Design review of the part built by this model. Coordinates are the model's own, in mm. Face numbers are marked on the shaded views. Coordinates: 2 decimals unless noted, no trailing zeros. Write each loop counter-clockwise with the first axis right and the second up, starting at its lowest first coordinate (ties: lowest second). Pieces come first, ordered by that corner, then holes. Notation, with made-up numbers: (-20.75, 82) - (10.25, 82) arc R14 ccw to (10.25, 102) - close; hole circle Ø5 at (87, 78). An arc over 180 degrees is marked (long way). Answer as CSV lines item,"result". Start each with the question number.
Q1. We need section C-C (y = 13). Write out the cut boundary in (x, z).
Q2. We need section A-A (x = -4). Write out the cut boundary in (y, z), plus the area to 3 significant figures.
Q3. We need section B-B (z = 45). Write out the cut boundary in (x, y), plus the area to 3 significant figures.
Q4. Clearance check with flat-ended pins moving along their axes: pin 1 (3.5 mm diameter, centred on y = 5, z = 31, fed in from -X); pin 2 (6.5 mm diameter, centred on x = -2, y = 14, fed in from +Z); pin 3 (0.9 mm diameter, centred on x = -11.5, y = 35.5, fed in from -Z). State where each tip first meets the part, or that it passes through.
Q5. We need section D-D (z = 13). Write out the cut boundary in (x, y).
Q6. Mouldability with a two-part tool opening along Z and no side actions: class the marked faces 1 and 2 as pulls with the +Z half, pulls with the -Z half, needs draft (parallel to the pull), parting line crosses it, or undercut.
Q7. For line 1 along Y through (x, z) = (-8.8, -31); line 2 along Z through (x, y) = (0, 38.1); line 3 along Z through (x, y) = (-2.75, 27), list the stretches that pass through material, from the lowest coordinate up. Write a range as [from, to].
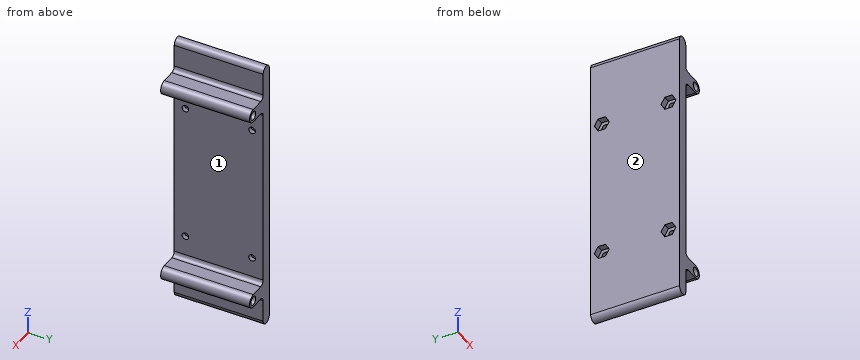
Autodesk Inventor part; units mm, degrees
ref_plane "РабПлоскость1" through (0, 20, 0) normal (0, 1, 0) x (1, 0, 0)
ref_plane "YZ Plane" through (0, 0, 0) normal (1, 0, 0) x (0, 1, 0)
ref_plane "XZ Plane" through (0, 0, 0) normal (0, 1, 0) x (-1, 0, 0)
sketch "Эскиз1" plane through (0, 0, 0) normal (0, 1, 0) x (-1, 0, 0)
  line L0 (0, 45) -> (0, -45) construction
  circle A0 centre (0, 45) radius 1.5
  circle A1 centre (0, -45) radius 1.5
  line L1 (10.5, 60) -> (10.5, -60) construction
  line L2 (10.5, -60) -> (10.5, 60) construction
  line L3 (13, -60) -> (13, 60)
  line L4 (8, 60) -> (8, 48)
  arc A2 (8, -60) -> (13, -60) centre (10.5, -60) ccw
  arc A3 (13, 60) -> (8, 60) centre (10.5, 60) ccw
  arc A4 (0, 42) -> (0, 48) centre (0, 45) ccw construction
  arc A5 (0, -48) -> (0, -42) centre (0, -45) ccw construction
  line L5 (0, 48) -> (8, 48)
  line L6 (0, 42) -> (8, 42)
  line L7 (0, -42) -> (8, -42)
  line L8 (0, -48) -> (8, -48)
  arc A6 (0, -42) -> (0, -48) centre (0, -45) ccw
  arc A7 (0, 48) -> (0, 42) centre (0, 45) ccw
  line L9 (8, -42) -> (8, -48) construction
  line L10 (8, 42) -> (8, -42)
  line L11 (8, -48) -> (8, -60)
  line L12 (8, 48) -> (8, 42) construction
  point P0 (0, 0)
  point P1 (0, 0)
  point P2 (10.5, 0)
  dimension "d0" = 90
  dimension "d1" = 3
  dimension "d2" = 3
  dimension "d3" = 120
  dimension "d4" = 10.5
  dimension "d5" = 0
  dimension "d6" = 5
  dimension "d7" = 6
  dimension "d8" = 6
extrude "Выдавливание1" add sketch "Эскиз1" along normal blind 40
fillet "Сопряжение1" radius 2 4 edges at (-8, 20, 42) (-8, 20, 48) (-8, 20, -42) (-8, 20, -48)
sketch "Эскиз2" plane through (0, 40, 0) normal (0, 1, 0) x (1, 0, 0)
  line L0 (0, 48) -> (-6, 48)
  arc A0 (-8, 50) -> (-6, 48) centre (-6, 50) ccw
  line L1 (-8, 50) -> (-8, 60)
  arc A1 (-8, 60) -> (-13, 60) centre (-10.5, 60) ccw
  line L2 (-13, 60) -> (-13, -60)
  arc A2 (-13, -60) -> (-8, -60) centre (-10.5, -60) ccw
  line L3 (-8, -60) -> (-8, -50)
  arc A3 (-6, -48) -> (-8, -50) centre (-6, -50) ccw
  line L4 (-6, -48) -> (0, -48)
  arc A4 (0, -48) -> (0, -42) centre (0, -45) ccw
  line L5 (0, -42) -> (-6, -42)
  arc A5 (-8, -40) -> (-6, -42) centre (-6, -40) ccw
  line L6 (-8, -40) -> (-8, 40)
  arc A6 (-6, 42) -> (-8, 40) centre (-6, 40) ccw
  line L7 (-6, 42) -> (0, 42)
  arc A7 (0, 42) -> (0, 48) centre (0, 45) ccw
  circle A8 centre (0, -45) radius 1.5
  circle A9 centre (0, 45) radius 1.5
  circle A10 centre (0, -45) radius 1.95
  circle A11 centre (0, 45) radius 1.95
  point P0 (0, 0)
  dimension "d12" = 3.9
  dimension "d13" = 3.9
extrude "Выдавливание2" cut sketch "Эскиз2" against normal blind 4 contours A8 | A9 | A10 | A11
ref_plane "РабПлоскость1" through (0, 20, 0) normal (0, 1, 0) x (1, 0, 0)
mirror "Зеркальное отражение1" about plane through (0, 20, 0) normal (0, 1, 0) of "Выдавливание2"
sketch "Эскиз3" plane through (-8, 0, 40) normal (1, 0, 0) x (0, 0, -1)
  line L0 (40, 0) -> (40, 40) construction
  line L1 (0, 40) -> (80, 40)
  line L2 (71, 5) -> (9, 5) construction
  line L3 (9, 5) -> (9, 35) construction
  line L4 (9, 35) -> (71, 35) construction
  line L5 (71, 35) -> (71, 5) construction
  line L6 (71, 5) -> (9, 35) construction
  line L7 (9, 5) -> (71, 35) construction
  circle A0 centre (9, 35) radius 1.5
  circle A1 centre (71, 35) radius 1.5
  circle A2 centre (9, 5) radius 1.5
  circle A3 centre (71, 5) radius 1.5
  point P0 (40, 20)
  dimension "d17" = 62
  dimension "d18" = 30
  dimension "d19" = 3
  dimension "d20" = 3
  dimension "d21" = 3
  dimension "d22" = 3
extrude "Выдавливание3" cut sketch "Эскиз3" against normal through all
sketch "Эскиз4" plane through (-13, 0, -60) normal (-1, 0, 0) x (0, 0, 1)
  circle A0 centre (29, 35) radius 1.5
  circle A1 centre (91, 35) radius 1.5
  line L0 (29, 35) -> (91, 35) construction
  circle A2 centre (91, 5) radius 1.5
  line L1 (91, 35) -> (91, 5) construction
  line L2 (91, 20) -> (60, 20) construction
  line L3 (60, 20) -> (60, 35) construction
  line L4 (31.9, 36.6743) -> (31.9, 33.3257)
  line L5 (31.9, 33.3257) -> (29, 31.6514)
  line L6 (29, 31.6514) -> (26.1, 33.3257)
  line L7 (26.1, 33.3257) -> (26.1, 36.6743)
  line L8 (26.1, 36.6743) -> (29, 38.3486)
  line L9 (29, 38.3486) -> (31.9, 36.6743)
  circle A3 centre (29, 5) radius 1.5
  line L10 (31.9, 3.3257) -> (31.9, 6.6743)
  line L11 (31.9, 6.6743) -> (29, 8.3486)
  line L12 (29, 8.3486) -> (26.1, 6.6743)
  line L13 (26.1, 6.6743) -> (26.1, 3.3257)
  line L14 (26.1, 3.3257) -> (29, 1.6514)
  line L15 (29, 1.6514) -> (31.9, 3.3257)
  line L16 (91, 38.3486) -> (93.9, 36.6743)
  line L17 (93.9, 36.6743) -> (93.9, 33.3257)
  line L18 (93.9, 33.3257) -> (91, 31.6514)
  line L19 (91, 31.6514) -> (88.1, 33.3257)
  line L20 (88.1, 33.3257) -> (88.1, 36.6743)
  line L21 (88.1, 36.6743) -> (91, 38.3486)
  circle A4 centre (91, 5) radius 1.5
  line L22 (91, 1.6514) -> (93.9, 3.3257)
  line L23 (93.9, 3.3257) -> (93.9, 6.6743)
  line L24 (93.9, 6.6743) -> (91, 8.3486)
  line L25 (91, 8.3486) -> (88.1, 6.6743)
  line L26 (88.1, 6.6743) -> (88.1, 3.3257)
  line L27 (88.1, 3.3257) -> (91, 1.6514)
  point P0 (60, 0)
  dimension "d25" = 31
  dimension "d26" = 5.8
  dimension "d27" = 5.8
  dimension "d28" = 5.8
  dimension "d29" = 5.8
extrude "Выдавливание4" cut sketch "Эскиз4" against normal blind 3 contours A0 | A1 | A2 | L4 L5 L6 L7 L8 L9 | A3 | L15 L14 L13 L12 L11 L10 | L16 L17 L18 L19 L20 L21 | L27 L26 L25 L24 L23 L22
equation "\"d8\" = d7"
properties part number "pod_akkum_2"
Results list:
1,outline,"(-13, -60) arc R2.5 ccw to (-8, -60) - (-8, -50) arc R2 cw to (-6, -48) - (0, -48) arc R3 ccw to (0, -42) - (-6, -42) arc R2 cw to (-8, -40) - (-8, 40) arc R2 cw to (-6, 42) - (0, 42) arc R3 ccw to (0, 48) - (-6, 48) arc R2 cw to (-8, 50) - (-8, 60) arc R2.5 ccw to (-13, 60) - close; hole circle Ø3 at (0, -45); hole circle Ø3 at (0, 45)"
2,outline,"(0, -48) - (40, -48) - (40, -42) - (0, -42) - close; (0, 42) - (40, 42) - (40, 48) - (0, 48) - close"
2,area,"480 mm2"
3,outline,"(-13, 0) - (-1.95, 0) - (-1.95, 4) - (-1.5, 4) - (-1.5, 36) - (-1.95, 36) - (-1.95, 40) - (-13, 40) - close; (1.5, 4) - (1.95, 4) - (1.95, 0) - (3, 0) - (3, 40) - (1.95, 40) - (1.95, 36) - (1.5, 36) - close"
3,area,"513 mm2"
4,pin 1,"stops at x = -10"
4,pin 2,"stops at z = 48"
4,pin 3,"stops at z = -62.44"
5,outline,"(-13, 0) - (-8, 0) - (-8, 40) - (-13, 40) - close"
6,face 1,"undercut"
6,face 2,"needs draft"
7,line 1,"y = [0, 3.5], [6.5, 33.5], [36.5, 40]"
7,line 2,"z = [-48, -46.95], [-43.05, -42], [42, 43.05], [46.95, 48]"
7,line 3,"z = [-48, -42], [42, 48]"
